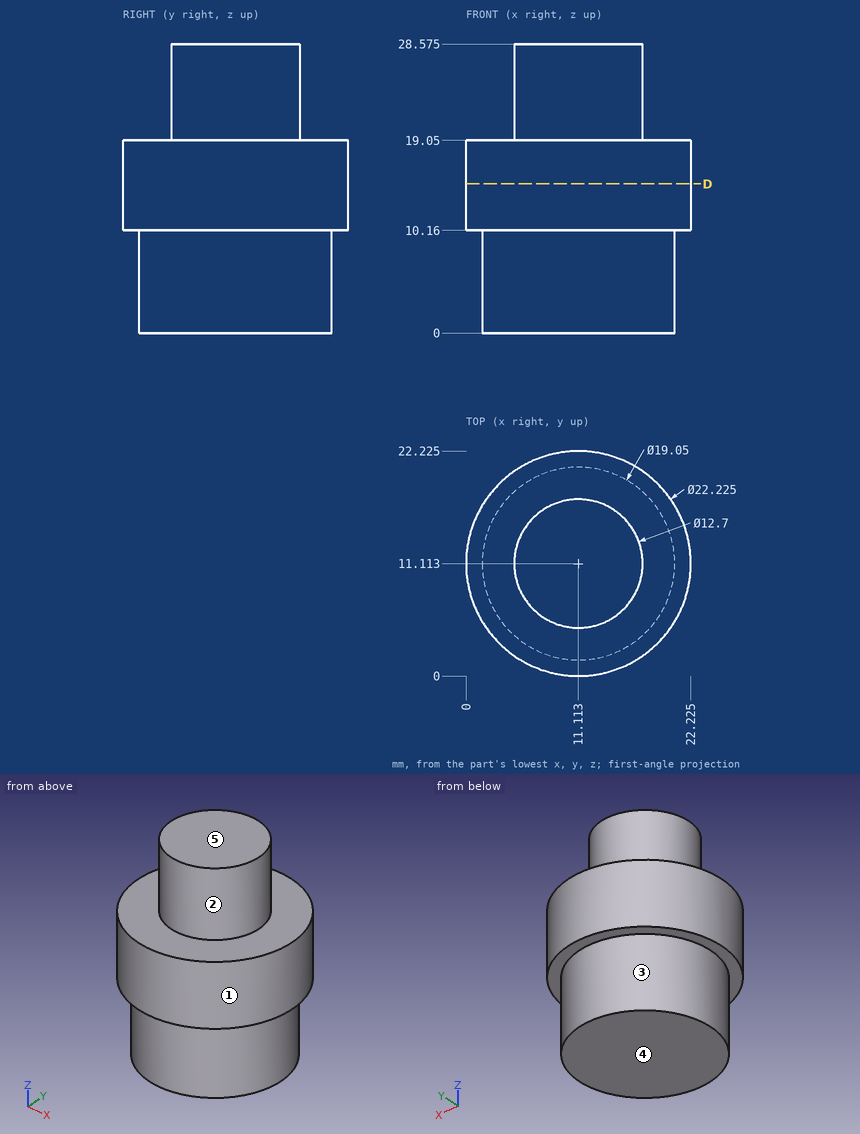
Check sheet for the drawn part. Datum: minimum x, y, z corner. Units: mm. A direction names the side the tool comes from. Give positions to 0.01 mm unless a question says otherwise; leave off trailing zeros. Order: outer loops, then holes, each group sorted by start corner. A loop starts at its lowest first (then second) coordinate and runs counter-clockwise, first axis right, second up. Notation, with made-up numbers: (18.5, 82) - (45.5, 82) arc R21 ccw to (45.5, 87) - close; hole circle Ø1 at (21.25, 48.5). An arc over 180 degrees is marked (long way). Write item = value, one per line. Start each with the question number.
1) Scan lines: L1, parallel to Z at x = 8.5, y = 19.25; L2, parallel to Z at x = 19, y = 3.5; L3, parallel to X at y = 11, z = 22.75. Record each from-to range of solid material in increasing order.
2) Section check D-D (z = 14.75). Enter the section's corners in (x, y) (1 decimal).
3) Draft check along Z on the marked faces 3, 4 and 5. Enter one of: released by +Z, released by -Z, zero draft, split by the parting line, or undercut.
4) Gauge pin test, flat ends, axial feed: pin 1 Ø1.5 at (y, z) = (16, 21.5) entering from -X (1 decimal); pin 2 Ø4 at (y, z) = (14, 6) entering from +X; pin 3 Ø4 at (y, z) = (4, 4.5) entering from +X. Record the tip position at first contact, or that the pin passes through.
5) Access from +Z, -Z, +X, -X, +Y, -Y to the whole of each face (thin tool, end or side, straight path). Record for the marked faces 1 and 2.
Geometry check:
q1.L1 = 0 to 19.05
q1.L2 = 10.16 to 19.05
q1.L3 = 4.76 to 17.46
q2.outline = circle Ø22.2 at (11.1, 11.1)
q3.face_3 = zero draft
q3.face_4 = released by -Z
q3.face_5 = released by +Z
q4.pin_1 = 6.3
q4.pin_2 = 20.6
q4.pin_3 = 19.15
q5.face_1 = +Z, -Z
q5.face_2 = +Z
